Read the model definition and answer for the solid it produces. Units are mm, in the model's axes. Face numbers are marked on the shaded views. A direction names the side the tool comes from. Coordinates: 2 decimals unless noted, no trailing zeros. Write each loop counter-clockwise with the first axis right and the second up, starting at its lowest first coordinate (ties: lowest second). Pieces come first, ordered by that corner, then holes.
1) Each of these flat-tipped pins is pushed along its axis until it touches: pin 1 Ø3.5 at (x, z) = (-0.5, 12) entering from +Y; pin 2 Ø12 at (y, z) = (-6, 7.5) entering from -X; pin 3 Ø6 at (x, z) = (3, -36.5) entering from +Y (3 decimals). Where does it stop, or does it pass through?
2) The part is cut by section C-C (z = 1.5). Determine the outline of the cut face in (x, y) (1 decimal).
3) The part is cut by section D-D (z = -38.5). Determine the outline of the cut face in (x, y) (3 decimals), then the cut area to 3 significant figures.
4) The part is cut by section A-A (y = 0). Determine the outline of the cut face in (x, z) (1 decimal).
5) The part is cut by section B-B (x = 0). Determine the outline of the cut face in (y, z) (1 decimal).
6) Find the intervals of material crossed by line 1 (Z direction, x = -8.5, y = 4.5); line 2 (Y direction, x = 0, z = 13.5); line 3 (Y direction, x = -10.5, z = -26), in increasing order.
7) Which of the six approach directions +Z, -Z, +X, -X, +Y, -Y give full straight-line access (tool end or side, diameter ignored) to the marked faces 1 and 2?
from build123d import *

# Parameters (mm, degrees)
SKETCH1_R           = 18.415
BOSS_EXTRUDE1_DEPTH = 55.88
SKETCH1_3_R         = 6.0325
BOSS_EXTRUDE2_DEPTH = 5.08
BOSS_EXTRUDE3_DEPTH = 15.494


with BuildPart() as part:
    # Sketch1 → Boss-Extrude1 (new body)
    with BuildSketch(Plane.XY):
        Circle(SKETCH1_R)
    extrude(amount=-BOSS_EXTRUDE1_DEPTH)

    # Sketch1<3> → Boss-Extrude2 (add)
    with BuildSketch(Plane.XY):
        Circle(SKETCH1_3_R)
    extrude(amount=BOSS_EXTRUDE2_DEPTH)

    # Sketch3 → Boss-Extrude3 (add)
    with BuildSketch(Plane.XY.offset(5.08)):
        with BuildLine():
            Line((-1.665589385, 2.4765), (1.665589385, 2.4765))
            ThreePointArc((1.665589385, 2.4765), (0, -2.9845), (-1.665589385, 2.4765))
        make_face()
    extrude(amount=BOSS_EXTRUDE3_DEPTH)


solid = part.part
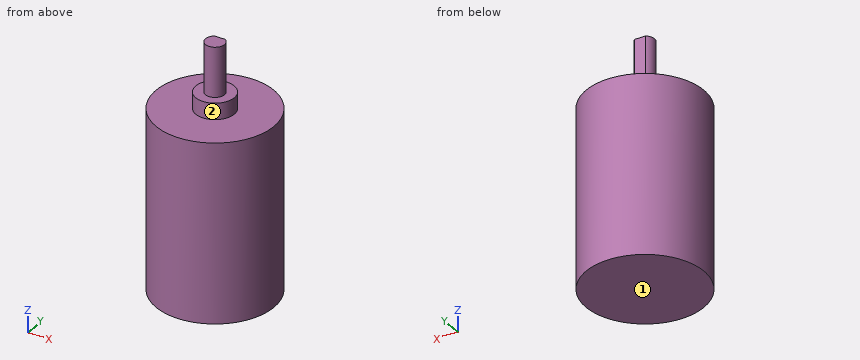
Reported:
1. pin 1: stops at y = 2.48
1. pin 2: stops at x = -6.01
1. pin 3: stops at y = 18.415
2. outline: circle Ø12.1 at (0, 0)
3. outline: circle Ø36.83 at (0, 0)
3. area: 1,070 mm2
4. outline: (-18.4, -55.9) - (18.4, -55.9) - (18.4, 0) - (6, 0) - (6, 5.1) - (3, 5.1) - (3, 20.6) - (-3, 20.6) - (-3, 5.1) - (-6, 5.1) - (-6, 0) - (-18.4, 0) - close
5. outline: (-18.4, -55.9) - (18.4, -55.9) - (18.4, 0) - (6, 0) - (6, 5.1) - (2.5, 5.1) - (2.5, 20.6) - (-3, 20.6) - (-3, 5.1) - (-6, 5.1) - (-6, 0) - (-18.4, 0) - close
6. line 1: z = -55.88 to 0
6. line 2: y = -2.98 to 2.48
6. line 3: y = -15.13 to 15.13
7. face 1: -Z, +X, -X, +Y, -Y
7. face 2: +Z
